from build123d import *

# Parameters (mm, degrees)
F2_DEPTH = 5
F3_R     = 62.5
F4_DEPTH = 25
F5_R     = 13.5
F6_DEPTH = 150


with BuildPart() as f1:
    # F0 (on Front) → F1 (revolve)
    with BuildSketch(Plane.XZ):
        with BuildLine():
            ThreePointArc((-15, 0), (-7.538172, 1.135519), (0, 1.515308))
            Line((0, 1.515308), (0, 190))
            Line((0, 190), (-15, 190))
            Line((-15, 190), (-15, 0))
        make_face()
    revolve(axis=Axis((0, 0, 81.138), (0, 0, -1)))

    # F0 (on Front) → F2 (join, symmetric)
    with BuildSketch(Plane.XZ):
        with BuildLine():
            Line((-15, 0), (0, 0))
            Line((0, 0), (0, 1.515308))
            ThreePointArc((0, 1.515308), (-7.538172, 1.135519), (-15, 0))
        make_face()
        with BuildLine():
            Line((0, 1.515308), (0, 0))
            Line((0, 0), (-15, 0))
            ThreePointArc((-15, 0), (-47.434165, -131.579442), (75, -73.484692))
            ThreePointArc((75, -73.484692), (53.033009, -20.451684), (0, 1.515308))
        make_face()
    extrude(amount=F2_DEPTH, both=True)

    # F3 (on face) → F4 (cut)
    with BuildSketch(Plane.XZ.offset(5)):
        with Locations((0, -73.484692)):
            Circle(F3_R)
    extrude(amount=-F4_DEPTH, mode=Mode.SUBTRACT)

    # F5 (on face) → F6 (cut)
    with BuildSketch(Plane.XY.offset(190)):
        Circle(F5_R)
    extrude(amount=-F6_DEPTH, mode=Mode.SUBTRACT)


solid = f1.part
Source: CAD feature listing. Evaluate the final solid. Frame: model axes, mm. A direction names the side the tool comes from. Coordinates: 2 decimals unless noted, no trailing zeros. Order: outer loops, then holes, each group sorted by start corner. A loop starts at its lowest first (then second) coordinate and runs counter-clockwise, first axis right, second up. Notation, with made-up numbers: M 88.5,50.25 L 130.5,50.25 A12 cw 130.5,66.25 Z; hole C 60,27.25 d6. An arc over 180 degrees is marked long. Write each question's results on one line, items separated by ' | '. Start each with the question number.
1. Pin query (flat end, axial travel): pin 1 (1.5 mm diameter, centred on y = -11, z = 77.5, fed in from +X); pin 2 (5 mm diameter, centred on y = 1.5, z = 63.5, fed in from -X); pin 3 (1.5 mm diameter, centred on y = 5.5, z = -95, fed in from -X). Return the tip coordinate at first contact, or that it passes through.
2. Section A-A, the plane z = -63. Return the cut outline in (x, y).
3. Section B-B, the plane x = -28. Return the cut outline in (y, z).
4. Material intervals for L1, parallel to Y at x = 0, z = 100; L2, parallel to Z at x = 0, y = 0; L3, parallel to Z at x = 48, y = 3, sorted ascending.
5. Draft query along X for faces 1 (the face through (14.985, 0.66, 93.67)), 2 (the face through (0, 0, 40)), 3 (the face through (-11.18, 7.85, 190)). Return one class per face: +X half, -X half, draft (parallel to the pull), parting line (faces both ways), or undercut.
6. Reachability of faces 4 (the face through (-2.93, -13.18, 116.05)), 5 (the face through (-13.55, -0.07, -134.5)) from +Z, -Z, +X, -X, +Y, -Y: full face, straight path, thin tool, end or side. Return the list, or none.
7. Section C-C, the plane z = 142. Return the cut outline in (x, y), then the cut area to 3 significant figures.
Solution:
1) pin 1: x = 10.95 | pin 2: x = -15 | pin 3: x = -72.01
2) outline: M -74.26,-5 L -61.61,-5 L -61.61,5 L -74.26,5 Z; M 61.61,-5 L 74.26,-5 L 74.26,5 L 61.61,5 Z
3) outline: M -5,-143.06 L 5,-143.06 L 5,-129.36 L -5,-129.36 Z; M -5,-17.61 L 5,-17.61 L 5,-3.91 L -5,-3.91 Z
4) L1: -15 to -13.5, 13.5 to 15 | L2: -148.48 to -135.98, -10.98 to 40 | L3: -131.11 to -113.51, -33.46 to -15.86
5) face 1: parting line | face 2: undercut | face 3: draft
6) face 4: +Z | face 5: +Y, -Y
7) outline: C 0,0 d30; hole C 0,0 d27 | area: 134 mm²
